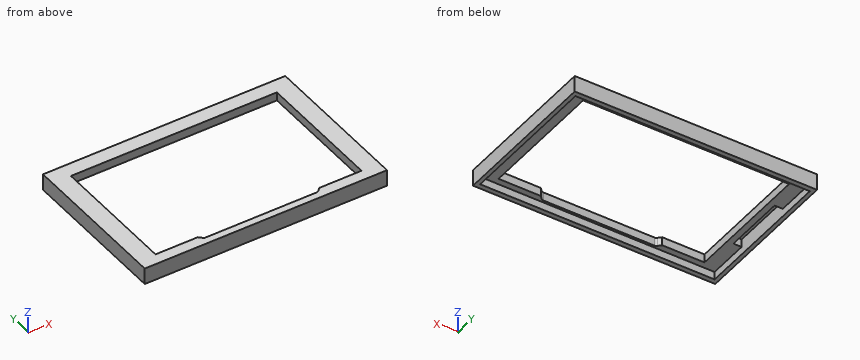
from build123d import *

# Parameters (mm, degrees)
SKETCH_W        = 74.1
SKETCH_H        = 47
PAD_DEPTH       = 5
SKETCH001_W     = 71.7
SKETCH001_H     = 44
POCKET_DEPTH    = 2.4
POCKET001_DEPTH = 5
SKETCH004_W     = 2.5
SKETCH004_H     = 19
POCKET002_DEPTH = 2.4
CHAMFER_SIZE    = 1.1
CHAMFER001_SIZE = 1.1
FILLET_R        = 1
FILLET001_R     = 1


with BuildPart() as part:
    # Sketch → Pad (new body)
    with BuildSketch(Plane.XY):
        Rectangle(SKETCH_W, SKETCH_H)
    extrude(amount=PAD_DEPTH)

    # Sketch001 (on Face5 of Pad) → Pocket (cut)
    with BuildSketch(Plane(origin=(0, 0, 0), x_dir=(1, 0, 0), z_dir=(0, 0, -1))):
        Rectangle(SKETCH001_W, SKETCH001_H)
    extrude(amount=-POCKET_DEPTH, mode=Mode.SUBTRACT)

    # Sketch002 (on Face5 of Pocket) → Pocket001 (cut)
    with BuildSketch(Plane.XY.offset(5)):
        Polygon((-31.5, 19), (31.5, 19), (31.5, -20.1), (18.5, -20.1), (18.5, -21.3), (-18.5, -21.3), (-18.5, -20.1), (-31.5, -20.1), align=None)
    extrude(amount=-POCKET001_DEPTH, mode=Mode.SUBTRACT)

    # Sketch004 (on Face19 of Pocket001) → Pocket002 (cut)
    with BuildSketch(Plane(origin=(0, 0, 2.4), x_dir=(1, 0, 0), z_dir=(0, 0, -1))):
        with Locations((-34.6, 0)):
            Rectangle(SKETCH004_W, SKETCH004_H)
    extrude(amount=-POCKET002_DEPTH, mode=Mode.SUBTRACT)

    # Chamfer
    chamfer_edges = [part.edges().sort_by_distance(p)[0] for p in [
        (-18.5, -21.3, 3.7),
    ]]
    chamfer(chamfer_edges, length=CHAMFER_SIZE)

    # Chamfer001
    chamfer001_edges = [part.edges().sort_by_distance(p)[0] for p in [
        (18.5, -21.3, 3.7),
    ]]
    chamfer(chamfer001_edges, length=CHAMFER001_SIZE)

    # Fillet
    fillet_edges = [part.edges().sort_by_distance(p)[0] for p in [
        (17.4, -21.3, 3.7),
    ]]
    fillet(fillet_edges, radius=FILLET_R)

    # Fillet001
    fillet001_edges = [part.edges().sort_by_distance(p)[0] for p in [
        (-17.4, -21.3, 3.7),
    ]]
    fillet(fillet001_edges, radius=FILLET001_R)


solid = part.part
Can you work these out from the model? Positions are in its coordinate system, mm. Coordinates: 2 decimals unless noted, no trailing zeros. Order: outer loops, then holes, each group sorted by start corner. A loop starts at its lowest first (then second) coordinate and runs counter-clockwise, first axis right, second up. Notation, with made-up numbers: M 52.25,0.25 L 109.25,0.25 A9 cw 109.25,16.25 Z; hole C 82,-17 d11. An arc over 180 degrees is marked long. Write item = value, one per line.
(1) Suppose I cut it at B-B on y = -11. Please give me the cut outline in (x, z).
Results are:
outline = M -37.05,0 L -35.85,0 L -35.85,2.4 L -31.5,2.4 L -31.5,5 L -37.05,5 Z; M 31.5,2.4 L 35.85,2.4 L 35.85,0 L 37.05,0 L 37.05,5 L 31.5,5 Z
(2) Suppose I cut it at C-C on z = 3.6. Please give me the cut outline in (x, y), plus the area to 3 significant figures.
Results are:
outline = M -37.05,-23.5 L 37.05,-23.5 L 37.05,23.5 L -37.05,23.5 Z; hole M -35.85,-9.5 L -33.35,-9.5 L -33.35,9.5 L -35.85,9.5 Z; hole M -31.5,-20.1 L -18.5,-20.1 L -18.5,-20.2 L -17.69,-21.01 A1 ccw -16.99,-21.3 L 16.99,-21.3 A1 ccw 17.69,-21.01 L 18.5,-20.2 L 18.5,-20.1 L 31.5,-20.1 L 31.5,19 L -31.5,19 Z
area = 929 mm2
(3) Suppose I cut it at A-A on x = 19.5. Please give me the cut outline in (y, z).
Results are:
outline = M -23.5,0 L -22,0 L -22,2.4 L -20.1,2.4 L -20.1,5 L -23.5,5 Z; M 19,2.4 L 22,2.4 L 22,0 L 23.5,0 L 23.5,5 L 19,5 Z
(4) Suppose I cut it at D-D on y = 8. Please give me the cut outline in (x, z), plus the area to 3 significant figures.
Results are:
outline = M -37.05,0 L -35.85,0 L -35.85,4.8 L -33.35,4.8 L -33.35,2.4 L -31.5,2.4 L -31.5,5 L -37.05,5 Z; M 31.5,2.4 L 35.85,2.4 L 35.85,0 L 37.05,0 L 37.05,5 L 31.5,5 Z
area = 28.6 mm2
(5) I need wall thicknesses on line 1 along X through (y, z) = (-2.5, 2.45); line 2 along Y through (x, z) = (-16.5, 4.6); line 3 along X through (y, z) = (-14, 4.5). Which ranges of each line are inside material? Lowest first, please. Write a range as [from, to].
Results are:
line_1 = [-37.05, -35.85], [-33.35, -31.5], [31.5, 37.05]
line_2 = [-23.5, -21.3], [19, 23.5]
line_3 = [-37.05, -31.5], [31.5, 37.05]
